```python
from build123d import *

# Parameters (mm, degrees)
F2_W     = 75
F2_H     = 50
F3_DEPTH = 19.5
F4_W     = 73
F4_H     = 45
F5_DEPTH = 18.5
F6_W     = 10
F6_H     = 4
F7_DEPTH = 1
F8_R     = 3.5
F9_DEPTH = 4


with BuildPart() as f3:
    # F2 (on Top) → F3 (new body)
    with BuildSketch(Plane.XY):
        Rectangle(F2_W, F2_H)
    extrude(amount=F3_DEPTH)

    # F4 (on face) → F5 (cut)
    with BuildSketch(Plane.XY.offset(19.5)):
        with Locations((0, -1.5)):
            Rectangle(F4_W, F4_H)
    extrude(amount=-F5_DEPTH, mode=Mode.SUBTRACT)

    # F6 (on face) → F7 (cut, through all)
    with BuildSketch(Plane.XZ.offset(25)):
        with Locations((0, 7.5)):
            Rectangle(F6_W, F6_H)
    extrude(amount=-F7_DEPTH, mode=Mode.SUBTRACT)

    # F8 (on face) → F9 (cut, through all)
    with BuildSketch(Plane(origin=(0, 25, 0), x_dir=(-1, 0, 0), z_dir=(0, 1, 0))):
        with Locations((-25, 8.5)):
            Circle(F8_R)
        with Locations((0, 8.5)):
            Circle(F8_R)
        with Locations((25, 8.5)):
            Circle(F8_R)
    extrude(amount=-F9_DEPTH, mode=Mode.SUBTRACT)


solid = f3.part
```
Build history of the part. All positions in model axes, mm. A direction names the side the tool comes from. Round coordinates to 2 decimals unless told otherwise and drop trailing zeros. Order: outer loops, then holes, each group sorted by start corner. A loop starts at its lowest first (then second) coordinate and runs counter-clockwise, first axis right, second up. Notation, with made-up numbers: (-1.75, 46.5) - (26.25, 46.5) arc R22 cw to (26.25, 83.5) - close; hole circle Ø10 at (-2.5, -37). An arc over 180 degrees is marked (long way). Use a Markdown table: item, result.
1) Saw through at D-D on z = 8.5. Write the cut outline in (x, y), and give its area (3 significant figures).
Recorded:
| item | result |
|---|---|
| outline | (-37.5, -25) - (-5, -25) - (-5, -24) - (-36.5, -24) - (-36.5, 21) - (-28.5, 21) - (-28.5, 25) - (-37.5, 25) - close; (-21.5, 21) - (-3.5, 21) - (-3.5, 25) - (-21.5, 25) - close; (3.5, 21) - (21.5, 21) - (21.5, 25) - (3.5, 25) - close; (5, -25) - (37.5, -25) - (37.5, 25) - (28.5, 25) - (28.5, 21) - (36.5, 21) - (36.5, -24) - (5, -24) - close |
| area | 371 mm² |
2) Tool access for faces 4 (the face through (-1, -24, 10)), 5 (the face through (37.5, 0, 10)), 6 (the face through (23.385, 23.028, 5.395)): list every direction of +Z, -Z, +X, -X, +Y, -Y with a clear straight run to the whole face (end or side of a thin tool).
Recorded:
| item | result |
|---|---|
| face 4 | +Z |
| face 5 | +Z, -Z, +X, +Y, -Y |
| face 6 | +Y |
3) Wall check: L1, parallel to Y at x = 27.5, z = 18.75; L2, parallel to X at y = -9.5, z = 9.5; L3, parallel to Z at x = 0, y = 22.45. Give the ranges that are in metal, low to high.
Recorded:
| item | result |
|---|---|
| L1 | y = -25 to -24, 21 to 25 |
| L2 | x = -37.5 to -36.5, 36.5 to 37.5 |
| L3 | z = 0 to 5, 12 to 19.5 |
4) Saw through at A-A on x = 25. Write the cut outline in (y, z).
Recorded:
| item | result |
|---|---|
| outline | (-25, 0) - (25, 0) - (25, 5) - (21, 5) - (21, 1) - (-24, 1) - (-24, 19.5) - (-25, 19.5) - close; (21, 12) - (25, 12) - (25, 19.5) - (21, 19.5) - close |
5) Saw through at B-B on z = 13.5. Write the cut outline in (x, y).
Recorded:
| item | result |
|---|---|
| outline | (-37.5, -25) - (37.5, -25) - (37.5, 25) - (-37.5, 25) - close; hole (-36.5, -24) - (36.5, -24) - (36.5, 21) - (-36.5, 21) - close |
6) Pull direction Y, two halves, no side cores. Call faces 1 (the face through (-37.5, 0, 10)), 2 (the face through (-36.5, -2, 10)), 3 (the face through (-1, -25, 10)): pulls with the +Y half, pulls with the -Y half, needs draft (parallel to the pull), parting line crosses it, or undercut.
Recorded:
| item | result |
|---|---|
| face 1 | needs draft |
| face 2 | undercut |
| face 3 | pulls with the -Y half |
7) Flat gauge pin, fed straight in: pin 1 Ø5 at (x, y) = (-14, 11) entering from +Z. Where does the tip first touch, or does it go through?
Recorded:
| item | result |
|---|---|
| pin 1 | stops at z = 1 |
8) Saw through at C-C on y = 5. Write the cut outline in (x, z).
Recorded:
| item | result |
|---|---|
| outline | (-37.5, 0) - (37.5, 0) - (37.5, 19.5) - (36.5, 19.5) - (36.5, 1) - (-36.5, 1) - (-36.5, 19.5) - (-37.5, 19.5) - close |
